Autodesk Fusion 360 part; units mm, degrees
sketch "Sketch1" plane through (0, 0, 0) normal (0, 0, 1) x (1, 0, 0)
  line L0 (0, 0) -> (139.7, 0)
  line L1 (139.7, 0) -> (139.7, 40)
  line L2 (139.7, 40) -> (0, 40)
  line L3 (0, 40) -> (0, 0)
  dimension "d1" = 139.7
  dimension "d2" = 40
extrude "Extrude1" add sketch "Sketch1" along normal blind 5
sketch "Sketch2" plane through (0, 0, 0) normal (0, 0, 1) x (1, 0, 0)
  point P0 (6.35, 20)
  point P1 (133.35, 20)
hole "Hole1" at (6.35, 20, 0) at (133.35, 20, 0) direction (0, 0, 1) diameter 5.5 depth 13 tip angle 118 counterbore diameter 9.1 counterbore depth 1
sketch "Sketch7" plane through (0, 0, 5) normal (0, 0, 1) x (-1, 0, 0)
  circle A0 centre (-6.35, -20) radius 2.75
  circle A1 centre (-133.35, -20) radius 2.75
  line L0 (0, -40) -> (0, 0)
  line L1 (0, 0) -> (-139.7, 0)
  line L2 (-139.7, 0) -> (-139.7, -40)
  line L3 (-139.7, -40) -> (0, -40)
  line L4 (-85.775, -40) -> (-123.775, -40)
  line L5 (-123.775, -40) -> (-123.775, 0)
  line L6 (-123.775, 0) -> (-85.775, 0)
  line L7 (-85.775, 0) -> (-85.775, -40)
  line L8 (-85.775, -40) -> (-123.775, 0) construction
  line L9 (-123.775, -40) -> (-85.775, 0) construction
  line L10 (-15.925, -40) -> (-53.925, -40)
  line L11 (-53.925, -40) -> (-53.925, 0)
  line L12 (-53.925, 0) -> (-15.925, 0)
  line L13 (-15.925, 0) -> (-15.925, -40)
  line L14 (-15.925, -40) -> (-53.925, 0) construction
  line L15 (-53.925, -40) -> (-15.925, 0) construction
  point P0 (-104.775, -20)
  point P1 (-34.925, -20)
  point P2 (-104.775, -20)
  point P3 (-34.925, -20)
  dimension "d25" = 38
  dimension "d26" = 40
  dimension "d27" = 38
  dimension "d28" = 40
extrude "Extrude4" add sketch "Sketch7" along normal blind 11 contours L1 L3 L10 L11 L12 L13 | L1 L3 L4 L5 L6 L7
sketch "Sketch8" plane through (0, 40, 0) normal (0, 1, 0) x (-1, 0, 0)
  line L0 (-139.7, 0) -> (0, 0)
  line L1 (0, 0) -> (0, 5)
  line L2 (0, 5) -> (-15.925, 5)
  line L3 (-15.925, 5) -> (-15.925, 16)
  line L4 (-15.925, 16) -> (-53.925, 16)
  line L5 (-53.925, 16) -> (-53.925, 5)
  line L6 (-53.925, 5) -> (-85.775, 5)
  line L7 (-85.775, 5) -> (-85.775, 16)
  line L8 (-85.775, 16) -> (-123.775, 16)
  line L9 (-123.775, 16) -> (-123.775, 5)
  line L10 (-123.775, 5) -> (-139.7, 5)
  line L11 (-139.7, 5) -> (-139.7, 0)
  circle A0 centre (-104.775, 16) radius 10
  circle A1 centre (-34.925, 16) radius 10
  point P0 (-104.775, 16)
  point P1 (-34.925, 16)
  dimension "d31" = 20
  dimension "d32" = 20
extrude "Extrude5" cut sketch "Sketch8" against normal blind 400 contours L8 A0 | L4 A1 picked at (-104.876, 11.6935) picked at (-35.1741, 12.676)
sketch "Sketch9" plane through (0, 0, 16) normal (0, 0, 1) x (-1, 0, 0)
  line L0 (-24.925, 0) -> (-24.925, -40)
  line L1 (-24.925, -40) -> (-15.925, -40)
  line L2 (-15.925, -40) -> (-15.925, 0)
  line L3 (-15.925, 0) -> (-24.925, 0)
  point P0 (-20.375, -5)
  point P1 (-20.375, -35)
  point P2 (-49.475, -5)
  point P3 (-49.475, -35)
  point P4 (-90.225, -35)
  point P5 (-90.225, -5)
  point P6 (-119.325, -35)
  point P7 (-119.325, -5)
hole "Hole4" at (20.375, 35, 16) at (20.375, 5, 16) at (49.475, 5, 16) at (49.475, 35, 16) at (90.225, 35, 16) at (90.225, 5, 16) at (119.325, 5, 16) at (119.325, 35, 16) direction (0, 0, -1) diameter 5.1 depth 11 tip angle 180
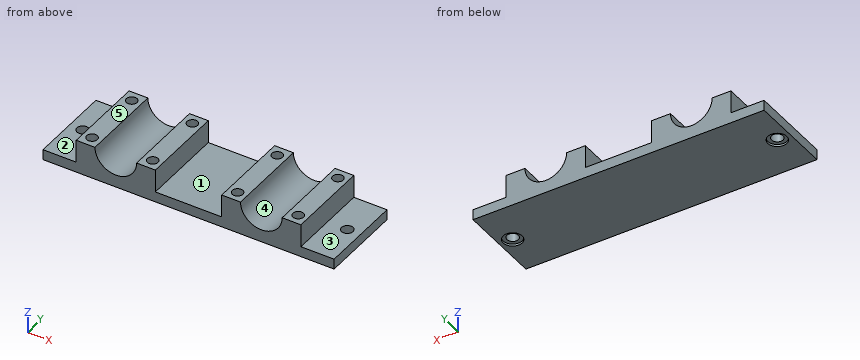
Input: part model. Units: mm. Frame: model coordinates. Face numbers are marked on the shaded views. A direction names the side the tool comes from. Coordinates: 2 decimals unless noted, no trailing zeros. Loops run counter-clockwise (first coordinate to the right, second up) from the corner with the lowest first, then second, coordinate; pieces in that order, holes last. Notation, with made-up numbers: (71, 37.25) - (88, 37.25) arc R25 ccw to (88, 63.25) - close; hole circle Ø7 at (42.25, 76.5). An arc over 180 degrees is marked (long way). Answer in a Markdown table with one row per item. Add a question column.
Item 1: Section query A-A on y = 20. State how many separate pieces and enclosed holes the cut face has, then the cut area to 3 significant figures.
Item 2: Section query B-B on x = 6.35. Return the cut outline in (y, z).
Item 3: Line query: line 1 along X through (y, z) = (20, 2); line 2 along X through (y, z) = (20, 0.5); line 3 along X through (y, z) = (12, 11) (3 decimals). Output: solid intervals per line, ascending. Write a range as [from, to].
Item 4: Contact query for flat-ended pins moving along their axis: P1, Ø8, axis at x = 6.35, y = 20, coming from the +Z side; P2, Ø6, axis at x = 32, y = 25.5, coming from the +Z side; P3, Ø4, axis at y = 32, z = 11.5, coming from the -X side (3 decimals); P4, Ø5, axis at x = 6.35, y = 20, coming from the -Z side. Output: stop coordinate, or through.
Item 5: Access query for the marked faces 1, 2 and 3. Directions: +Z, -Z, +X, -X, +Y, -Y. A direction counts if a zero-diameter tool reaches every point of the face in a straight line with its end or side. Return the directions, or none.
Item 6: Mould query, pull axis X, two halves, no side actions, for the marked faces 4 and 5. Classes: released by +X, released by -X, zero draft, split by the parting line, or undercut.
Recorded:
| question | item | result |
|---|---|---|
| 1 | separate pieces | 3 |
| 1 | enclosed holes | 0 |
| 1 | area | 1,160 mm^2 |
| 2 | outline | (0, 0) - (15.45, 0) - (15.45, 1) - (17.25, 1) - (17.25, 5) - (0, 5) - close; (22.75, 1) - (24.55, 1) - (24.55, 0) - (40, 0) - (40, 5) - (22.75, 5) - close |
| 3 | line 1 | [0, 3.6], [9.1, 130.6], [136.1, 139.7] |
| 3 | line 2 | [0, 1.8], [10.9, 128.8], [137.9, 139.7] |
| 3 | line 3 | [15.925, 26.265], [43.585, 53.925], [85.775, 96.115], [113.435, 123.775] |
| 4 | P1 | z = 5 |
| 4 | P2 | z = 7.94 |
| 4 | P3 | x = 15.925 |
| 4 | P4 | through |
| 5 | face 1 | +Z, +Y, -Y |
| 5 | face 2 | +Z, -X, +Y, -Y |
| 5 | face 3 | +Z, +X, +Y, -Y |
| 6 | face 4 | undercut |
| 6 | face 5 | zero draft |
